```python
from build123d import *

# Parameters (mm, degrees)
F0_W     = 450
F0_H     = 476
F1_DEPTH = 8
F3_DEPTH = 16.001
F4_W     = 4
F4_H     = 5
F5_DEPTH = 450.001


# Not quite as in the source:
# - a feature names something its author has since deleted; it is built from what else it names


with BuildPart() as f1:
    # F0 (on Top) → F1 (new body, symmetric)
    with BuildSketch(Plane.XY):
        Rectangle(F0_W, F0_H)
    extrude(amount=F1_DEPTH, both=True)

    # F2 (on face) → F3 (cut, through all)
    with BuildSketch(Plane.XY.offset(8)):
        with BuildLine():
            ThreePointArc((149.9904602378, 220.9366969629), (140.0025066822, 230.4999996858), (130.0097599498, 220.9417054897))
            ThreePointArc((130.0097599498, 220.9417054897), (139.5607987599, 210.5096495421), (149.9904602378, 220.0633030371))
            Line((149.9904602378, 220.0633030371), (149.9904602378, 220.9366969629))
        make_face()
        with BuildLine():
            Line((149.9904602378, 220.9366969629), (149.9904602378, 220.0633030371))
            ThreePointArc((149.9904602378, 220.0633030371), (149.997614775, 220.2815994251), (150, 220.5))
            ThreePointArc((150, 220.5), (149.997614775, 220.7184005749), (149.9904602378, 220.9366969629))
        make_face()
        with BuildLine():
            Line((130.0097599498, 238), (130.0097599498, 220.9417054897))
            ThreePointArc((130.0097599498, 220.9417054897), (140.0025066822, 230.4999996858), (149.9904602378, 220.9366969629))
            Line((149.9904602378, 220.9366969629), (149.9904602378, 238))
            Line((149.9904602378, 238), (130.0097599498, 238))
        make_face()
    extrude(amount=-F3_DEPTH, mode=Mode.SUBTRACT)

    # F4 (on face) → F5 (cut, through all)
    with BuildSketch(Plane.YZ.offset(225)):
        with Locations((-228, 5.5)):
            Rectangle(F4_W, F4_H)
    extrude(amount=-F5_DEPTH, mode=Mode.SUBTRACT)


solid = f1.part
```
The model under review builds one solid part; all positions refer to its coordinate system, in mm. A direction names the side the tool comes from. Coordinates: 2 decimals unless noted, no trailing zeros. Order: outer loops, then holes, each group sorted by start corner. A loop starts at its lowest first (then second) coordinate and runs counter-clockwise, first axis right, second up. Notation, with made-up numbers: (-24.75, 33.25) -> (-2.75, 33.25) arc R17 cw to (-2.75, 60.25) -> close; hole circle Ø3 at (7, 84.25). An arc over 180 degrees is marked (long way). Answer in a Markdown table with one row per item. Add a question column.
Item 1: To check wall thickness, follow probe 1 along Y at (x, z) = (47, 4.25); probe 2 along Y at (x, z) = (132, 6). State the ranges of each line that lie inside material, in increasing order.
Item 2: Mouldability with a two-part tool opening along X and no side actions: class faces 3 (the flat face through (-3, 9, 8)), 4 (the flat face through (225, -3, 0)), 5 (the flat face through (149.99, 229, 0)) as +X half, -X half, draft (parallel to the pull), parting line (faces both ways), or undercut.
Item 3: Machinability: for faces 1 (the flat face through (130.01, 230, 0)), 2 (the flat face through (-3, 3, -8)), which of the approach directions +Z, -Z, +X, -X, +Y, -Y give a long, thin tool a straight path to every point of the face, cutting with its end or side? Answer none if there is none.
Item 4: We need section A-A on x = 140. Write out the cut boundary in (y, z), plus the area to 3 significant figures.
Final values:
| question | item | result |
|---|---|---|
| 1 | probe 1 | y = -238 to -230, -226 to 238 |
| 1 | probe 2 | y = -238 to -230, -226 to 214.5 |
| 2 | face 3 | draft |
| 2 | face 4 | +X half |
| 2 | face 5 | undercut |
| 3 | face 1 | +Z, -Z, +Y |
| 3 | face 2 | -Z, +X, -X, +Y, -Y |
| 4 | outline | (-238, -8) -> (210.5, -8) -> (210.5, 8) -> (-226, 8) -> (-226, 3) -> (-230, 3) -> (-230, 8) -> (-238, 8) -> close |
| 4 | area | 7,160 mm2 |
